Input: part model. Units: mm. Frame: model coordinates. Face numbers are marked on the shaded views. A direction names the side the tool comes from. Give positions to 0.01 mm unless a question says otherwise; leave off trailing zeros. Order: outer loops, then holes, each group sorted by start corner. A loop starts at its lowest first (then second) coordinate and runs counter-clockwise, first axis right, second up. Notation, with made-up numbers: (61.5, 82) - (97.5, 82) arc R11 ccw to (97.5, 98) - close; hole circle Ø4 at (71, -4). An arc over 180 degrees is marked (long way). Answer in a Markdown table with one row per item. Add a question column.
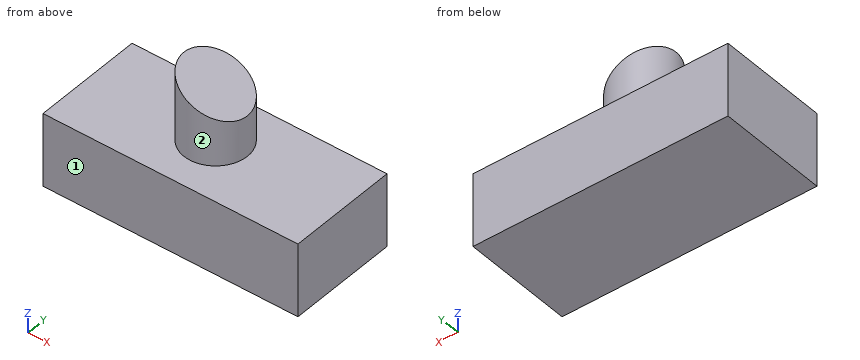
from build123d import *

# Parameters (mm, degrees)
F0_W     = 88.247977
F0_H     = 38.269773
F1_DEPTH = 25.4
F2_R     = 10.984207
F3_DEPTH = 25.4
F5_DEPTH = 25.4
F6_DEPTH = 25.4


with BuildPart() as f1:
    # F0 (on Top) → F1 (new body)
    with BuildSketch(Plane.XY):
        with Locations((0.800162, -1.280717)):
            Rectangle(F0_W, F0_H)
    extrude(amount=F1_DEPTH)

    # F2 (on face) → F3 (join)
    with BuildSketch(Plane.XY.offset(25.4)):
        Circle(F2_R)
    extrude(amount=F3_DEPTH)

    # F4 (on Front) → F5 (cut)
    with BuildSketch(Plane.XZ):
        Polygon((19.144135, 55.871744), (-14.150013, 55.871744), (-18.519871, 54.207034), (19.144135, 35.479076), align=None)
    extrude(amount=-F5_DEPTH, mode=Mode.SUBTRACT)

    # F4 (on Front) → F6 (cut)
    with BuildSketch(Plane.XZ):
        Polygon((19.144135, 55.871744), (-14.150013, 55.871744), (-18.519871, 54.207034), (19.144135, 35.479076), align=None)
    extrude(amount=F6_DEPTH, mode=Mode.SUBTRACT)


solid = f1.part
Q1. Contact query for flat-ended pins moving along their axis: P1, Ø4, axis at x = -23.5, y = -6.5, coming from the +Z side; P2, Ø8, axis at x = 6, z = 35.5, coming from the +Y side; P3, Ø3, axis at y = -13, z = 44.5, coming from the +X side; P4, Ø1, axis at x = 27.5, y = 9.5, coming from the -Z side. Output: stop coordinate, or through.
Q2. Section D-D, the plane y = -18. Return loops of the section in (x, z), then the cut area to 3 significant figures.
Q3. Section C-C, the plane z = 38. Return loops of the section in (x, y), then the cut area to 3 significant figures.
Q4. Access query for the marked faces 1 and 2. Directions: +Z, -Z, +X, -X, +Y, -Y. A direction counts if a zero-diameter tool reaches every point of the face in a straight line with its end or side. Return the directions, or none.
Q5. Section A-A, the plane y = 0. Return loops of the section in (x, z), then the cut area to 3 significant figures.
Q6. Section B-B, the plane x = 0. Return loops of the section in (y, z).
Q7. Line query: probe 1 along Z at (x, y) = (-34, 1); probe 2 along X at (y, z) = (-3, 41.5); probe 3 along Z at (x, y) = (-1.5, 8.5). Output: solid intervals per line, ascending.
Computed:
| question | item | result |
|---|---|---|
| 1 | P1 | stops at z = 25.4 |
| 1 | P2 | stops at y = 10.8 |
| 1 | P3 | passes through |
| 1 | P4 | stops at z = 0 |
| 2 | outline | (-43.32, 0) - (44.92, 0) - (44.92, 25.4) - (-43.32, 25.4) - close |
| 2 | area | 2,240 mm^2 |
| 3 | outline | circle Ø21.97 at (0, 0) |
| 3 | area | 379 mm^2 |
| 4 | face 1 | +Z, -Z, +X, -X, -Y |
| 4 | face 2 | +Z |
| 5 | outline | (-43.32, 0) - (44.92, 0) - (44.92, 25.4) - (10.98, 25.4) - (10.98, 39.54) - (-10.98, 50.46) - (-10.98, 25.4) - (-43.32, 25.4) - close |
| 5 | area | 2,670 mm^2 |
| 6 | outline | (-20.42, 0) - (17.85, 0) - (17.85, 25.4) - (10.98, 25.4) - (10.98, 45) - (-10.98, 45) - (-10.98, 25.4) - (-20.42, 25.4) - close |
| 7 | probe 1 | z = 0 to 25.4 |
| 7 | probe 2 | x = -10.57 to 7.04 |
| 7 | probe 3 | z = 0 to 45.74 |
